Part model, mm, in its own coordinate system. Give positions to 0.01 mm unless a question says otherwise; leave off trailing zeros. Order: outer loops, then holes, each group sorted by start corner. A loop starts at its lowest first (then second) coordinate and runs counter-clockwise, first axis right, second up.
1. Slice it at A-A on y = 1.4. List the corners of the cut face in (x, z).
2. Slice it at C-C on z = 242.5. List the corners of the cut face in (x, y), and give its area (3 significant figures).
3. Drop flat-ended pins along their axis: pin 1 Ø0.7 at (x, y) = (-281, 1) entering from +Z; pin 2 Ø1.1 at (y, z) = (1, -301.5) entering from -X; pin 3 Ø0.7 at (x, y) = (308, 0.5) entering from -Z. Give the stop position or say it passes through.
4. Slice it at B-B on x = -236.5. List the corners of the cut face in (y, z), and give its area (3 significant figures).
5. Probe line 1 (Z direction, x = -237.5, y = 1.3); line 2 (X direction, y = 0.9, z = 238.5); line 3 (Z direction, x = 250.5, y = 0.7). List the from-to ranges inside material, lowest first.
from build123d import *
from OCP.BRepAlgoAPI import BRepAlgoAPI_Cut
from OCP.TopTools import TopTools_ListOfShape

# Parameters (mm, degrees)
SKETCH1_W           = 711.2
SKETCH1_H           = 711.2
BOSS_EXTRUDE1_DEPTH = 2.252762246
SKETCH2_W           = 139.700021816
SKETCH2_H           = 139.700021816
CUT_EXTRUDE2_DEPTH  = 67.238084533
SKETCH3_W           = 140.054303581
SKETCH3_H           = 140.080522497
CUT_EXTRUDE3_DEPTH  = 67.238084533
SKETCH4_W           = 138.94158885
SKETCH4_H           = 138.94158885
CUT_EXTRUDE4_DEPTH  = 67.238084533
SKETCH5_W           = 139.27145682
SKETCH5_H           = 139.336797366
CUT_EXTRUDE5_DEPTH  = 67.238084533


with BuildPart() as part:
    # Sketch1 → Boss-Extrude1 (new body)
    with BuildSketch(Plane(origin=(0, 0, 0), x_dir=(1, 0, 0), z_dir=(0, 1, 0))):
        Rectangle(SKETCH1_W, SKETCH1_H)
    extrude(amount=BOSS_EXTRUDE1_DEPTH)


with BuildPart() as cut_extrude2_tool:
    # Sketch2 → Cut-Extrude2 (new body)
    with BuildSketch(Plane.XZ):
        with Locations((-285.749998801, 285.749986662)):
            Rectangle(SKETCH2_W, SKETCH2_H)
    extrude(amount=-CUT_EXTRUDE2_DEPTH)


with BuildPart() as part_1:
    add(part.part)

    # Cut-Extrude2: cut by cut_extrude2_tool, with a tolerance
    cut_extrude2_stock = TopTools_ListOfShape()
    cut_extrude2_stock.Append(part_1.part.wrapped)
    cut_extrude2_tools = TopTools_ListOfShape()
    cut_extrude2_tools.Append(cut_extrude2_tool.part.wrapped)
    cut_extrude2_cut = BRepAlgoAPI_Cut()
    cut_extrude2_cut.SetArguments(cut_extrude2_stock)
    cut_extrude2_cut.SetTools(cut_extrude2_tools)
    cut_extrude2_cut.SetFuzzyValue(0.00001)
    cut_extrude2_cut.Build()
    add(Compound.cast(cut_extrude2_cut.Shape()).solids(), mode=Mode.REPLACE)

    # Sketch3 → Cut-Extrude3 (cut)
    with BuildSketch(Plane(origin=(0, 2.252762246, 0), x_dir=(1, 0, 0), z_dir=(0, 1, 0))):
        with Locations((285.57284821, -285.559738752)):
            Rectangle(SKETCH3_W, SKETCH3_H)
    extrude(amount=-CUT_EXTRUDE3_DEPTH, mode=Mode.SUBTRACT)

    # Sketch4 → Cut-Extrude4 (cut)
    with BuildSketch(Plane(origin=(0, 2.252762246, 0), x_dir=(1, 0, 0), z_dir=(0, 1, 0))):
        with Locations((-286.129205575, 286.129205575)):
            Rectangle(SKETCH4_W, SKETCH4_H)
    extrude(amount=-CUT_EXTRUDE4_DEPTH, mode=Mode.SUBTRACT)

    # Sketch5 → Cut-Extrude5 (cut)
    with BuildSketch(Plane(origin=(0, 2.252762246, 0), x_dir=(1, 0, 0), z_dir=(0, 1, 0))):
        with Locations((285.96427159, 285.931601317)):
            Rectangle(SKETCH5_W, SKETCH5_H)
    extrude(amount=-CUT_EXTRUDE5_DEPTH, mode=Mode.SUBTRACT)


solid = part_1.part
Data:
1. outline: (-355.6, -216.66) - (-216.66, -216.66) - (-216.66, -355.6) - (216.33, -355.6) - (216.33, -216.26) - (355.6, -216.26) - (355.6, 215.52) - (215.55, 215.52) - (215.55, 355.6) - (-215.9, 355.6) - (-215.9, 215.9) - (-355.6, 215.9) - close
2. outline: (-215.9, 0) - (215.55, 0) - (215.55, 2.25) - (-215.9, 2.25) - close
2. area: 972 mm2
3. pin 1: stops at z = 215.9
3. pin 2: stops at x = -216.66
3. pin 3: stops at z = -216.26
4. outline: (0, -216.66) - (2.25, -216.66) - (2.25, 215.9) - (0, 215.9) - close
4. area: 974 mm2
5. line 1: z = -216.66 to 215.9
5. line 2: x = -215.9 to 215.55
5. line 3: z = -216.26 to 215.52
